```python
from build123d import *

# Parameters (mm, degrees)
SKETCH1_W           = 25
SKETCH1_H           = 25
BOSS_EXTRUDE1_DEPTH = 120
CUT_EXTRUDE1_DEPTH  = 120
SKETCH3_W           = 25
SKETCH3_H           = 12.5
CUT_EXTRUDE2_DEPTH  = 120
FILLET1_R           = 2.5
FILLET2_R           = 2.5
FILLET3_R           = 2.5
SKETCH6_R           = 2.75
CUT_EXTRUDE3_DEPTH  = 10
SKETCH7_W           = 10.05
SKETCH7_H           = 15.1
CUT_EXTRUDE4_DEPTH  = 2.5


with BuildPart() as part:
    # Sketch1 → Boss-Extrude1 (new body)
    with BuildSketch(Plane(origin=(0, 0, 0), x_dir=(1, 0, 0), z_dir=(0, 1, 0))):
        Rectangle(SKETCH1_W, SKETCH1_H)
    extrude(amount=BOSS_EXTRUDE1_DEPTH)

    # Sketch2 → Cut-Extrude1 (cut)
    with BuildSketch(Plane(origin=(0, 120, 0), x_dir=(1, 0, 0), z_dir=(0, 1, 0))):
        Polygon((-10.25, -2.48824277), (-10.25, -10.25), (-2.61175723, -10.25), (-2.61175723, -5.15), (2.48824277, -5.15), (2.48824277, -10.25), (10.25, -10.25), (10.25, -2.61175723), (5.15, -2.61175723), (5.15, 2.48824277), (10.25, 2.48824277), (10.25, 10.25), (2.61175723, 10.25), (2.61175723, 5.15), (-2.48824277, 5.15), (-2.48824277, 10.25), (-10.25, 10.25), (-10.25, 2.61175723), (-5.15, 2.61175723), (-5.15, -2.48824277), align=None)
    extrude(amount=-CUT_EXTRUDE1_DEPTH, mode=Mode.SUBTRACT)

    # Sketch3 → Cut-Extrude2 (cut)
    with BuildSketch(Plane(origin=(0, 120, 0), x_dir=(1, 0, 0), z_dir=(0, 1, 0))):
        with Locations((0, 6.25)):
            Rectangle(SKETCH3_W, SKETCH3_H)
    extrude(amount=-CUT_EXTRUDE2_DEPTH, mode=Mode.SUBTRACT)

    # Fillet1
    fillet1_edges = [part.edges().sort_by_distance(p)[0] for p in [
        (-12.5, 60, 0),
    ]]
    fillet(fillet1_edges, radius=FILLET1_R)

    # Fillet2
    fillet2_edges = [part.edges().sort_by_distance(p)[0] for p in [
        (12.5, 60, 0),
    ]]
    fillet(fillet2_edges, radius=FILLET2_R)

    # Fillet3
    # the kernel refuses this fillet: 2.5 mm, written as the material it takes off along each edge
    with BuildSketch(Plane(origin=(-10, 0, 0), x_dir=(0, 0, 1), z_dir=(1, 0, 0)), Plane(origin=(-1.1, 0, 0), x_dir=(0, 0, 1), z_dir=(1, 0, 0)), Plane(origin=(-10, 120, 0), x_dir=(0, -1, 0), z_dir=(1, 0, 0)), Plane(origin=(-1.1, 120, 0), x_dir=(0, -1, 0), z_dir=(1, 0, 0))) as fillet3_piece_1:
        with BuildLine():
            CenterArc((FILLET3_R, -FILLET3_R), FILLET3_R, 90, 90)
            Line((0, -FILLET3_R), (0, 0))
            Line((0, 0), (FILLET3_R, 0))
        make_face()
    extrude(amount=11.1, mode=Mode.SUBTRACT)
    with BuildSketch(Plane(origin=(-10, 0, 2.5), x_dir=(-1, 0, 0), z_dir=(0, 0, 1))) as fillet3_piece_2:
        with BuildLine():
            CenterArc((2.5 - FILLET3_R, -FILLET3_R), FILLET3_R, 0, 90)
            Line((2.5, -FILLET3_R), (2.5, 0))
            Line((2.5, 0), (2.5 - FILLET3_R, 0))
        make_face()
    revolve(axis=Axis((-10, 0, 2.5), (0, -1, 0)), revolution_arc=90, mode=Mode.SUBTRACT)
    with BuildSketch(Plane(origin=(10, 0, 2.5), x_dir=(1, 0, 0), z_dir=(0, 0, 1))) as fillet3_piece_3:
        with BuildLine():
            CenterArc((2.5 - FILLET3_R, FILLET3_R), FILLET3_R, 270, 90)
            Line((2.5, FILLET3_R), (2.5, 0))
            Line((2.5, 0), (2.5 - FILLET3_R, 0))
        make_face()
    revolve(axis=Axis((10, 0, 2.5), (0, 1, 0)), revolution_arc=90, mode=Mode.SUBTRACT)
    with BuildSketch(Plane(origin=(-10, 120, 2.5), x_dir=(-1, 0, 0), z_dir=(0, 0, 1))) as fillet3_piece_4:
        with BuildLine():
            CenterArc((2.5 - FILLET3_R, FILLET3_R), FILLET3_R, 270, 90)
            Line((2.5 - FILLET3_R, 0), (2.5, 0))
            Line((2.5, 0), (2.5, FILLET3_R))
        make_face()
    revolve(axis=Axis((-10, 120, 2.5), (0, -1, 0)), revolution_arc=90, mode=Mode.SUBTRACT)
    with BuildSketch(Plane(origin=(10, 120, 2.5), x_dir=(1, 0, 0), z_dir=(0, 0, 1))) as fillet3_piece_5:
        with BuildLine():
            CenterArc((2.5 - FILLET3_R, -FILLET3_R), FILLET3_R, 0, 90)
            Line((2.5 - FILLET3_R, 0), (2.5, 0))
            Line((2.5, 0), (2.5, -FILLET3_R))
        make_face()
    revolve(axis=Axis((10, 120, 2.5), (0, 1, 0)), revolution_arc=90, mode=Mode.SUBTRACT)
    with BuildSketch(Plane(origin=(-18.75, 0, 12.5), x_dir=(0, 0, -1), z_dir=(1, 0, 0)), Plane(origin=(-18.75, 120, 12.5), x_dir=(0, -1, 0), z_dir=(1, 0, 0))) as fillet3_piece_6:
        with BuildLine():
            CenterArc((FILLET3_R, FILLET3_R), FILLET3_R, 180, 90)
            Line((0, FILLET3_R), (0, 0))
            Line((0, 0), (FILLET3_R, 0))
        make_face()
    extrude(amount=37.5, mode=Mode.SUBTRACT)
    with BuildSketch(Plane(origin=(-12.5, 0, 2.5), x_dir=(1, 0, 0), z_dir=(0, 0, 1)), Plane(origin=(12.5, 0, 18.75), x_dir=(-1, 0, 0), z_dir=(0, 0, -1)), Plane(origin=(-12.5, 120, 2.5), x_dir=(0, -1, 0), z_dir=(0, 0, 1)), Plane(origin=(12.5, 120, 18.75), x_dir=(0, -1, 0), z_dir=(0, 0, -1))) as fillet3_piece_7:
        with BuildLine():
            CenterArc((FILLET3_R, FILLET3_R), FILLET3_R, 180, 90)
            Line((0, FILLET3_R), (0, 0))
            Line((0, 0), (FILLET3_R, 0))
        make_face()
    extrude(amount=16.25, mode=Mode.SUBTRACT)

    # Sketch6 → Cut-Extrude3 (cut)
    with BuildSketch(Plane.XY.offset(12.5)):
        with Locations((0, 107.5)):
            Circle(SKETCH6_R)
        with Locations((0, 12.5)):
            Circle(SKETCH6_R)
    extrude(amount=-CUT_EXTRUDE3_DEPTH, mode=Mode.SUBTRACT)

    # Sketch7 → Cut-Extrude4 (cut)
    with BuildSketch(Plane(origin=(0, 0, 5.15), x_dir=(-1, 0, 0), z_dir=(0, 0, -1))):
        with Locations((0, 107.5)):
            Rectangle(SKETCH7_W, SKETCH7_H)
        with Locations((0, 12.5)):
            Rectangle(SKETCH7_W, SKETCH7_H)
    extrude(amount=-CUT_EXTRUDE4_DEPTH, mode=Mode.SUBTRACT)


solid = part.part
```
The listing builds one solid part. Answer for the finished solid, in the listing's coordinates (mm). A direction names the side the tool comes from. Give positions to 0.01 mm unless a question says otherwise; leave off trailing zeros. Loops run counter-clockwise (first coordinate to the right, second up) from the corner with the lowest first, then second, coordinate; pieces in that order, holes last. Notation, with made-up numbers: (75.5, 64) - (110.5, 64) arc R8 ccw to (110.5, 72) - close; hole circle Ø10 at (32.5, 5). An arc over 180 degrees is marked (long way). Answer as CSV lines item,"result". Start each with the question number.
Item 1: A cutting plane is placed at C-C on x = 7.5. Determine the outline of the cut face in (y, z), then the cut area to 3 significant figures.
Item 2: A cutting plane is placed at A-A on z = 8.75. Determine the outline of the cut face in (x, y), then the cut area to 3 significant figures.
Item 3: A cutting plane is placed at D-D on y = 72.5. Determine the outline of the cut face in (x, z), then the cut area to 3 significant figures.
Item 4: The mould has two halves that part along X. Classify faces 1 (the face through (0, 1, 12)), 2 (the face through (-12, 119, 7)), 3 (the face through (0, 112, 7.65)), 4 (the face through (0, 4.95, 6)): +X half, -X half, draft (parallel to the pull), parting line (faces both ways), or undercut.
Item 5: Find the intervals of material crossed by line 1 (Y direction, x = -0.25, z = 7.5); line 2 (Y direction, x = 0, z = 10.4); line 3 (X direction, y = 102.5, z = 7.75), in increasing order. Write a range as from..to.
Item 6: Each of these flat-tipped pins is pushed along its axis until it touches: pin 1 (2 mm diameter, centred on y = 65.5, z = 1, fed in from +X); pin 2 (9 mm diameter, centred on x = 0, y = 107.5, fed in from -Z); pin 3 (2.5 mm diameter, centred on x = 0, y = 1.5, fed in from -Z). Where does it stop, or does it pass through?
Item 7: A cutting plane is placed at B-B on x = 0. Determine the outline of the cut face in (y, z).
Item 8: For faces 5 (the face through (-6, 61, 10.25)), 6 (the face through (0, 20.05, 6)), 7 (the face through (2.488, 61, 8)), determine the directions among +Z, -Z, +X, -X, +Y, -Y from which every point of the face is accessible in a straight line to the end or side of a thin tool.
Found:
1,outline,"(0, 2.5) arc R2.5 ccw to (2.5, 0) - (117.5, 0) arc R2.5 ccw to (120, 2.5) - (120, 2.61) - (0, 2.61) - close; (0.01, 10.25) - (119.99, 10.25) arc R2.5 ccw to (117.5, 12.5) - (2.5, 12.5) arc R2.5 ccw to start"
1,area,"578 mm^2"
2,outline,"(-12.5, 2.5) arc R2.5 ccw to (-10.25, 0.01) - (-10.25, 119.99) arc R2.5 ccw to (-12.5, 117.5) - close; (-2.61, 0) - (2.49, 0) - (2.49, 11.33) arc R2.75 cw to (-2.61, 11.64) - close; (-2.61, 13.36) arc R2.75 cw to (2.49, 13.67) - (2.49, 106.33) arc R2.75 cw to (-2.61, 106.64) - close; (-2.61, 108.36) arc R2.75 cw to (2.49, 108.67) - (2.49, 120) - (-2.61, 120) - close; (10.25, 0.01) arc R2.5 ccw to (12.5, 2.5) - (12.5, 117.5) arc R2.5 ccw to (10.25, 119.99) - close"
2,area,"1,100 mm^2"
3,outline,"(-12.5, 2.5) arc R2.5 ccw to (-10, 0) - (-5.15, 0) - (-5.15, 2.49) - (-10.25, 2.49) - (-10.25, 10.25) - (-2.61, 10.25) - (-2.61, 5.15) - (2.49, 5.15) - (2.49, 10.25) - (10.25, 10.25) - (10.25, 2.61) - (5.15, 2.61) - (5.15, 0) - (10, 0) arc R2.5 ccw to (12.5, 2.5) - (12.5, 12.5) - (-12.5, 12.5) - close"
3,area,"152 mm^2"
4,face 1,"draft"
4,face 2,"-X half"
4,face 3,"undercut"
4,face 4,"undercut"
5,line 1,"y = 0..4.95, 20.05..99.95, 115.05..120"
5,line 2,"y = 0.03..9.75, 15.25..104.75, 110.25..119.97"
5,line 3,"x = -12.5..-10.25, -2.61..2.49, 10.25..12.5"
6,pin 1,"stops at x = 12.45"
6,pin 2,"stops at z = 7.65"
6,pin 3,"stops at z = 5.15"
7,outline,"(0, 5.15) - (4.95, 5.15) - (4.95, 7.65) - (9.75, 7.65) - (9.75, 12.5) - (2.5, 12.5) arc R2.5 ccw to (0, 10) - close; (15.25, 7.65) - (20.05, 7.65) - (20.05, 5.15) - (99.95, 5.15) - (99.95, 7.65) - (104.75, 7.65) - (104.75, 12.5) - (15.25, 12.5) - close; (110.25, 7.65) - (115.05, 7.65) - (115.05, 5.15) - (120, 5.15) - (120, 10) arc R2.5 ccw to (117.5, 12.5) - (110.25, 12.5) - close"
8,face 5,"+Y, -Y"
8,face 6,"-Z"
8,face 7,"-Z, +Y, -Y"
